Can you work these out from the drawing? Everything is in mm from the part's minimum corner. Give positions to 0.01 mm unless a question says otherwise; leave off trailing zeros. Write each loop counter-clockwise with the first axis right and the second up, starting at its lowest first coordinate (ties: lowest second). Pieces come first, ordered by that corner, then holes. Notation, with made-up numbers: (22.25, -0.75) - (53.25, -0.75) arc R29 ccw to (53.25, 34.25) - close; hole circle Ø8 at (-6.75, 40). An arc over 180 degrees is marked (long way). Use a Markdown table: item, result. Add a question column.
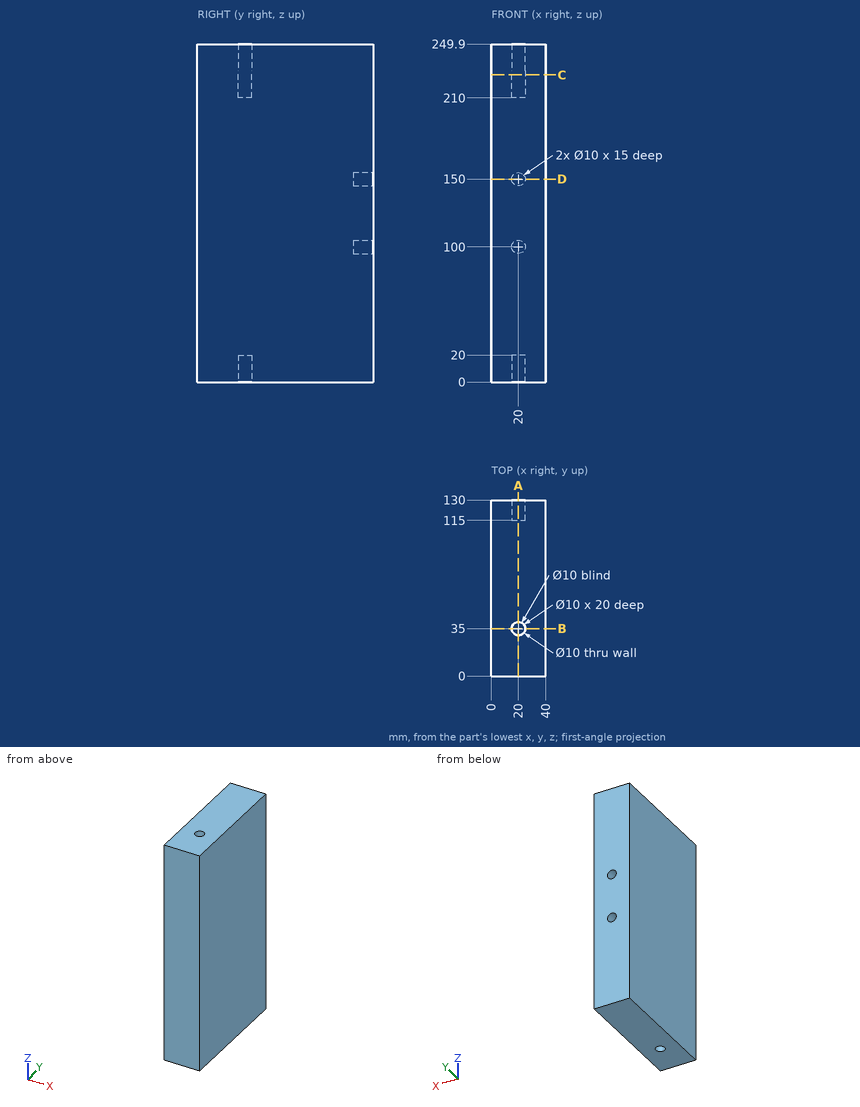
Q1. If I drill on probe 1 along Z at (x, y) = (20, 125.5); probe 2 along X at (y, z) = (35, 15.25); probe 3 along Y at (x, z) = (20, 225.5), over which ranges is the centre line in solid material (lowest first)? Write a range as [from, to].
Q2. Suppose I cut it at C-C (z = 227). Please give me the cut outline in (x, y), and give its area (3 significant figures).
Q3. Suppose I cut it at B-B (y = 35). Please give me the cut outline in (x, z).
Q4. Suppose I cut it at A-A (x = 20). Please give me the cut outline in (y, z), and give its area (3 significant figures).
Q5. Suppose I cut it at D-D (z = 150). Please give me the cut outline in (x, y).
Q6. I'm going to push flat-ended pins straight in: P1, Ø6, axis at x = 20, z = 100, coming from the +Y side; P2, Ø5, axis at x = 19, y = 35.5, coming from the +Z side; P3, Ø8, axis at x = 20, y = 33, coming from the -Z side; P4, Ø9, axis at x = 20, y = 35, coming from the -Z side. Where does each tip first touch, or does it pass through?
Derived:
| question | item | result |
|---|---|---|
| 1 | probe 1 | [0, 95], [105, 145], [155, 249.9] |
| 1 | probe 2 | [0, 15], [25, 40] |
| 1 | probe 3 | [0, 30], [40, 130] |
| 2 | outline | (0, 0) - (40, 0) - (40, 130) - (0, 130) - close; hole circle Ø10 at (20, 35) |
| 2 | area | 5,120 mm² |
| 3 | outline | (0, 0) - (15, 0) - (15, 20) - (25, 20) - (25, 0) - (40, 0) - (40, 249.9) - (25, 249.9) - (25, 210) - (15, 210) - (15, 249.9) - (0, 249.9) - close |
| 4 | outline | (0, 0) - (30, 0) - (30, 20) - (40, 20) - (40, 0) - (130, 0) - (130, 95) - (115, 95) - (115, 105) - (130, 105) - (130, 145) - (115, 145) - (115, 155) - (130, 155) - (130, 249.9) - (40, 249.9) - (40, 210) - (30, 210) - (30, 249.9) - (0, 249.9) - close |
| 4 | area | 31,600 mm² |
| 5 | outline | (0, 0) - (40, 0) - (40, 130) - (25, 130) - (25, 115) - (15, 115) - (15, 130) - (0, 130) - close |
| 6 | P1 | y = 115 |
| 6 | P2 | z = 210 |
| 6 | P3 | z = 0 |
| 6 | P4 | z = 20 |
